Design review of the part built by this model. Coordinates are the model's own, in mm. Face numbers are marked on the shaded views. Round coordinates to 2 decimals unless told otherwise and drop trailing zeros. Order: outer loops, then holes, each group sorted by start corner. A loop starts at its lowest first (then second) coordinate and runs counter-clockwise, first axis right, second up. Notation, with made-up numbers: (-6.75, 13.25) - (49.25, 13.25) arc R13 ccw to (49.25, 18.25) - close; hole circle Ø1 at (-7.75, 80). An arc over 180 degrees is marked (long way). Use CSV: the item, a comma, the result in double quotes.
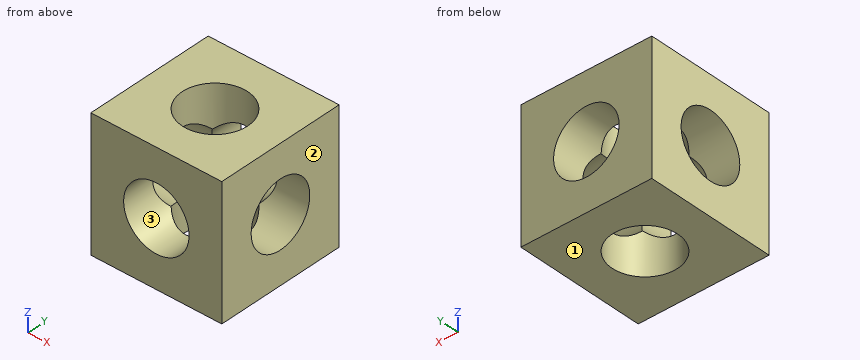
from build123d import *

# Parameters (mm, degrees)
F0_W     = 50
F0_H     = 50
F1_DEPTH = 50
F2_R     = 12.5
F3_DEPTH = 50
F4_R     = 12.5
F5_DEPTH = 50
F6_R     = 12.5
F7_DEPTH = 50


with BuildPart() as f1:
    # F0 (on Top) → F1 (new body)
    with BuildSketch(Plane.XY):
        Rectangle(F0_W, F0_H)
    extrude(amount=F1_DEPTH)

    # F2 (on face) → F3 (cut)
    with BuildSketch(Plane.XY.offset(50)):
        Circle(F2_R)
    extrude(amount=-F3_DEPTH, mode=Mode.SUBTRACT)

    # F4 (on face) → F5 (cut)
    with BuildSketch(Plane(origin=(-25, 0, 0), x_dir=(0, -1, 0), z_dir=(-1, 0, 0))):
        with Locations((0, 25)):
            Circle(F4_R)
    extrude(amount=-F5_DEPTH, mode=Mode.SUBTRACT)

    # F6 (on face) → F7 (cut)
    with BuildSketch(Plane(origin=(0, 25, 0), x_dir=(-1, 0, 0), z_dir=(0, 1, 0))):
        with Locations((0, 25)):
            Circle(F6_R)
    extrude(amount=-F7_DEPTH, mode=Mode.SUBTRACT)


solid = f1.part
1) We need section C-C (x = -14). Give the boundary of the cut face in (y, z).
Data:
outline,"(-25, 0) - (25, 0) - (25, 50) - (-25, 50) - close; hole circle Ø25 at (0, 25)"
2) We need section A-A (y = 7.5). Give the boundary of the cut face in (x, z).
Data:
outline,"(-25, 0) - (-10, 0) - (-10, 15) - (-25, 15) - close; (-25, 35) - (-10, 35) - (-10, 50) - (-25, 50) - close; (10, 0) - (25, 0) - (25, 15) - (10, 15) - close; (10, 35) - (25, 35) - (25, 50) - (10, 50) - close"
3) We need section B-B (z = 25). Give the boundary of the cut face in (x, y).
Data:
outline,"(-25, -25) - (-12.5, -25) - (-12.5, -12.5) - (-25, -12.5) - close; (-25, 12.5) - (-12.5, 12.5) - (-12.5, 25) - (-25, 25) - close; (12.5, -25) - (25, -25) - (25, -12.5) - (12.5, -12.5) - close; (12.5, 12.5) - (25, 12.5) - (25, 25) - (12.5, 25) - close"
4) To check wall thickness, follow L1, parallel to X at y = -20, z = 25; L2, parallel to Z at x = 21, y = 0; L3, parallel to Y at x = 0.5, z = 4.5. State the ranges of each line that lie inside material, in increasing order. Write a range as from..to.
Data:
L1,"x = -25..-12.5, 12.5..25"
L2,"z = 0..12.5, 37.5..50"
L3,"y = -25..-12.49, 12.49..25"
5) The part is to be moulded in two halves that separate along X. For the marked faces 1, 2 and 3, say which applies: +X half, -X half, draft (parallel to the pull), parting line (faces both ways), or undercut.
Data:
face 1,"draft"
face 2,"+X half"
face 3,"undercut"
